Input: part model. Units: mm. Frame: model coordinates. Face numbers are marked on the shaded views. A direction names the side the tool comes from. Give positions to 0.01 mm unless a question says otherwise; leave off trailing zeros. Loops run counter-clockwise (first coordinate to the right, second up) from the corner with the lowest first, then second, coordinate; pieces in that order, holes last. Notation, with made-up numbers: (72, -5) - (111, -5) arc R9 cw to (111, 2) - close; hole circle Ø6 at (1.25, -0.75). An arc over 180 degrees is marked (long way). Answer as a JSON object with one key per item and string values.
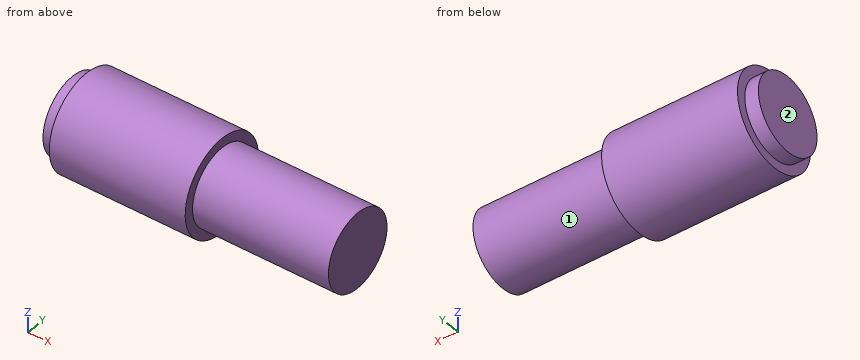
from build123d import *

# Parameters (mm, degrees)
SKETCH1_R           = 1.75
BOSS_EXTRUDE1_DEPTH = 5
SKETCH2_R           = 1.4
BOSS_EXTRUDE2_DEPTH = 10
SKETCH2_2_R         = 1.4
BOSS_EXTRUDE3_DEPTH = 0.5


with BuildPart() as part:
    # Sketch1 → Boss-Extrude1 (new body)
    with BuildSketch(Plane(origin=(0, 0, 0), x_dir=(0, 0, -1), z_dir=(1, 0, 0))):
        Circle(SKETCH1_R)
    extrude(amount=BOSS_EXTRUDE1_DEPTH)

    # Sketch2 → Boss-Extrude2 (add)
    with BuildSketch(Plane.ZY):
        Circle(SKETCH2_R)
    extrude(amount=-BOSS_EXTRUDE2_DEPTH)

    # Sketch2_2 → Boss-Extrude3 (add)
    with BuildSketch(Plane.ZY):
        Circle(SKETCH2_2_R)
    extrude(amount=BOSS_EXTRUDE3_DEPTH)


solid = part.part
Item 1: Cut plane C-C (x = 3.5). Return loops of the section in (y, z), then the cut area to 3 significant figures.
Geometry check:
{"outline": "circle Ø3.5 at (0, 0)", "area": "9.62 mm2"}
Item 2: Cut plane B-B (z = 0.25). Return loops of the section in (x, y), then the cut area to 3 significant figures.
Geometry check:
{"outline": "(-0.5, -1.38) - (0, -1.38) - (0, -1.73) - (5, -1.73) - (5, -1.38) - (10, -1.38) - (10, 1.38) - (5, 1.38) - (5, 1.73) - (0, 1.73) - (0, 1.38) - (-0.5, 1.38) - close", "area": "32.5 mm2"}
Item 3: Access query for the marked faces 1 and 2. Directions: +Z, -Z, +X, -X, +Y, -Y. A direction counts if a zero-diameter tool reaches every point of the face in a straight line with its end or side. Return the directions, or none.
Geometry check:
{"face 1": "+X", "face 2": "+Z, -Z, -X, +Y, -Y"}
Item 4: Cut plane A-A (y = 0). Return loops of the section in (x, z).
Geometry check:
{"outline": "(-0.5, -1.4) - (0, -1.4) - (0, -1.75) - (5, -1.75) - (5, -1.4) - (10, -1.4) - (10, 1.4) - (5, 1.4) - (5, 1.75) - (0, 1.75) - (0, 1.4) - (-0.5, 1.4) - close"}
Item 5: Material intervals for line 1 (X direction, y = -0.05, z = 1.55); line 2 (Y direction, x = 6, z = 0.3); line 3 (Y direction, x = 4.5, z = 0.5), sorted ascending. Write a range as [from, to].
Geometry check:
{"line 1": "x = [0, 5]", "line 2": "y = [-1.37, 1.37]", "line 3": "y = [-1.68, 1.68]"}
Item 6: Cut plane D-D (x = 6). Return loops of the section in (y, z).
Geometry check:
{"outline": "circle Ø2.8 at (0, 0)"}
Item 7: Contact query for flat-ended pins moving along their axis: P1, Ø1.5, axis at x = 8, y = 1.5, coming from the +Z side; P2, Ø2, axis at x = 8.5, y = 1.5, coming from the +Z side. Output: stop coordinate, or through.
Geometry check:
{"P1": "stops at z = 1.18", "P2": "stops at z = 1.31"}
